Drawing for the job (mm, zero at the part's lowest x, y, z). A direction names the side the tool comes from. Give positions to 0.01 mm unless a question says otherwise; leave off trailing zeros. Order: outer loops, then holes, each group sorted by start corner. A loop starts at its lowest first (then second) coordinate and runs counter-clockwise, first axis right, second up. Notation, with made-up numbers: M -11,-29 L 37,-29 A23 cw 37,-17 Z; hole C -5.5,68.25 d8. An arc over 180 degrees is marked long. Answer as a JSON object with one key per item and string values.
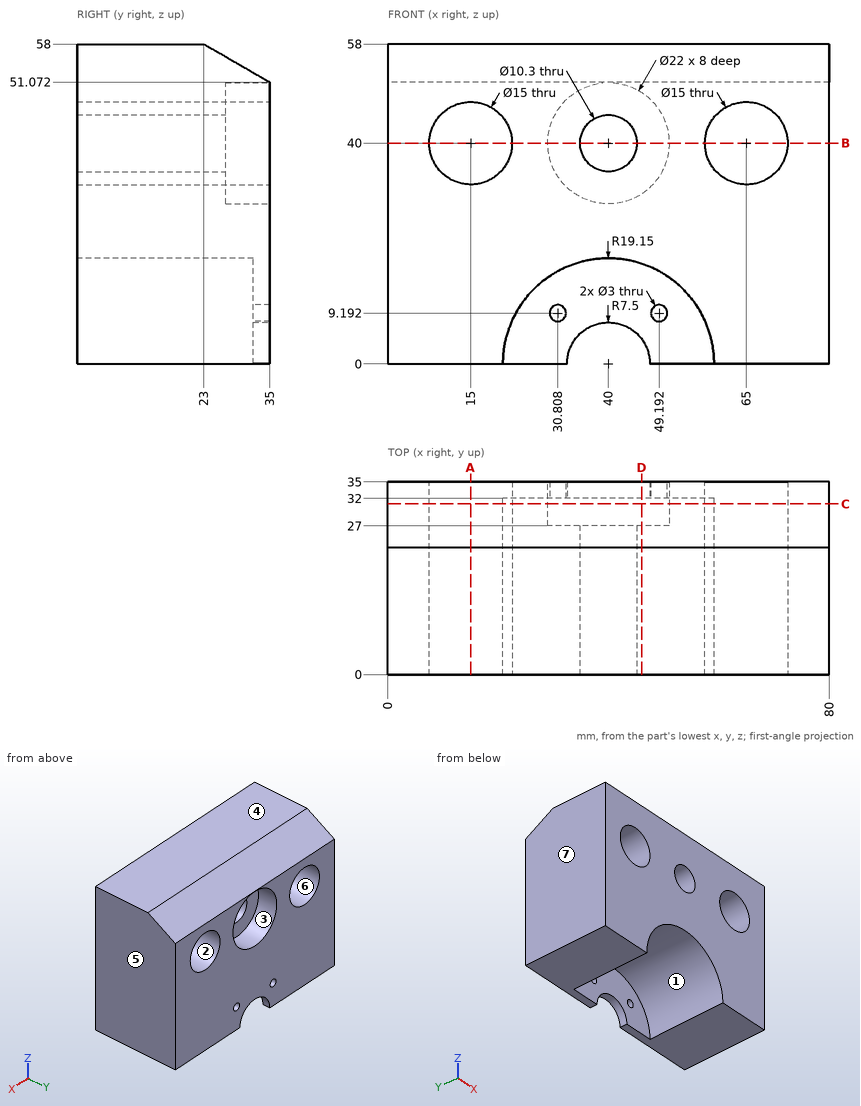
1. Cut at C-C on y = 31. Give the cut face in (x, z).
Worked answers:
{"outline": "M 0,0 L 20.85,0 A19.15 cw 59.15,0 L 80,0 L 80,53.38 L 0,53.38 Z; hole C 15,40 d15; hole C 40,40 d22; hole C 65,40 d15"}
2. Cut at D-D on x = 46. Give the cut face in (y, z) (1 decimal), plus the area to 3 significant figures.
Worked answers:
{"outline": "M 0,18.2 L 32,18.2 L 32,4.5 L 35,4.5 L 35,30.8 L 27,30.8 L 27,49.2 L 35,49.2 L 35,51.1 L 23,58 L 0,58 Z", "area": "1,250 mm^2"}
3. Cut at B-B on z = 40. Give the cut face in (x, y).
Worked answers:
{"outline": "M 0,0 L 7.5,0 L 7.5,35 L 0,35 Z; M 22.5,0 L 34.85,0 L 34.85,27 L 29,27 L 29,35 L 22.5,35 Z; M 45.15,0 L 57.5,0 L 57.5,35 L 51,35 L 51,27 L 45.15,27 Z; M 72.5,0 L 80,0 L 80,35 L 72.5,35 Z"}
4. Pin check, flat tips, straight feed: P1, Ø1.5, axis at x = 28, z = 44, coming from the -Y side; P2, Ø4, axis at x = 55.5, y = 29.5, coming from the +Z side; P3, Ø9.5, axis at x = 40, z = 11.5, coming from the -Y side; P4, Ø2, axis at x = 26, y = 29, coming from the +Z side. Stop position of each tip, or through.
Worked answers:
{"P1": "stops at y = 0", "P2": "stops at z = 55.4", "P3": "stops at y = 32", "P4": "stops at z = 55.11"}
5. Which spindle directions (+Z, -Z, +X, -X, +Y, -Y) get a long thin tool onto all of the face, cutting with end or side? Do the marked faces 1, 2 and 3. Say none if no direction does.
Worked answers:
{"face 1": "-Z, -Y", "face 2": "+Y, -Y", "face 3": "+Y"}
6. Probe line 1 along X through (y, z) = (24, 40); line 2 along X through (y, z) = (28.5, 40); line 3 along Z through (x, y) = (40, 16). List the from-to ranges inside material, lowest first.
Worked answers:
{"line 1": "x = 0 to 7.5, 22.5 to 34.85, 45.15 to 57.5, 72.5 to 80", "line 2": "x = 0 to 7.5, 22.5 to 29, 51 to 57.5, 72.5 to 80", "line 3": "z = 19.15 to 34.85, 45.15 to 58"}
7. Cut at A-A on x = 15. Give the cut face in (y, z).
Worked answers:
{"outline": "M 0,0 L 35,0 L 35,32.5 L 0,32.5 Z; M 0,47.5 L 35,47.5 L 35,51.07 L 23,58 L 0,58 Z"}
8. Two-plate mould, pull along X, no slides. Class the marked faces 4, 5, 6 and 7: +X half, -X half, draft (parallel to the pull), parting line (faces both ways), or undercut.
Worked answers:
{"face 4": "draft", "face 5": "+X half", "face 6": "undercut", "face 7": "-X half"}
